Geometry: final body of the model. Coordinates: model frame, mm. Give positions to 0.01 mm unless a question says otherwise; leave off trailing zeros. Write each loop counter-clockwise with the first axis right and the second up, starting at its lowest first coordinate (ties: lowest second). Pieces come first, ordered by that corner, then holes.
Q1. Line query: line 1 (X direction, y = 0.15, z = -15); line 2 (X direction, y = -0.25, z = -17.25); line 3 (Z direction, x = 0.5, y = -0.05). Output: solid intervals per line, ascending.
Q2. Section C-C (y = -0.15). Return the cut outline in (x, z), plus the area to 3 significant figures.
Q3. Section A-A (x = 0). Return the cut outline in (y, z).
Q4. Section B-B (z = -17.5). Return the cut outline in (x, y), plus the area to 3 significant figures.
Q5. Mould query, pull axis Z, two halves, no side actions, for faces 1 (the cylindrical face through (0.16, -0.08, 7.5)), 2 (the flat face through (0, -1, -8)), 3 (the cylindrical face through (0.931, -0.083, 2.957)). Classes: +Z half, -Z half, draft (parallel to the pull), parting line (faces both ways), or undercut.
Q6. Section D-D (z = -2). Return the cut outline in (x, y).
from build123d import *

# Parameters (mm, degrees)
BOSS_EXTRUDE1_DEPTH      = 0.86
BOSS_EXTRUDE1_DEPTH_BACK = 1
SKETCH1_R                = 3.1


with BuildPart() as part:
    # Sketch1 → Boss-Extrude1 (new, two sides: drawn at the far end of the back side and taken through both)
    with BuildSketch(Plane(origin=(0, 0, 0), x_dir=(1, 0, 0), z_dir=(0, 1, 0)).offset(-BOSS_EXTRUDE1_DEPTH_BACK)):
        with BuildLine():
            Line((-7.5, 0), (-7.5, 15))
            ThreePointArc((-7.5, 15), (0, 22.5), (7.5, 15))
            Line((7.5, 15), (7.5, 0))
            ThreePointArc((7.5, 0), (0, -7.5), (-7.5, 0))
        make_face()
        with Locations(Location((0, 0, 0), (0, 0, 270))):
            Circle(SKETCH1_R, mode=Mode.SUBTRACT)
        with Locations(Location((0, 15, 0), (0, 0, 270))):
            Circle(SKETCH1_R, mode=Mode.SUBTRACT)
    extrude(amount=BOSS_EXTRUDE1_DEPTH + BOSS_EXTRUDE1_DEPTH_BACK)


solid = part.part
Computed:
1. line 1: x = -7.5 to -3.1, 3.1 to 7.5
1. line 2: x = -7.15 to -2.13, 2.13 to 7.15
1. line 3: z = -22.48 to -18.06, -11.94 to -3.06, 3.06 to 7.48
2. outline: (-7.5, -15) arc R7.5 ccw to (7.5, -15) - (7.5, 0) arc R7.5 ccw to (-7.5, 0) - close; hole circle Ø6.2 at (0, -15); hole circle Ø6.2 at (0, 0)
2. area: 341 mm2
3. outline: (-1, -22.5) - (0.86, -22.5) - (0.86, -18.1) - (-1, -18.1) - close; (-1, -11.9) - (0.86, -11.9) - (0.86, -3.1) - (-1, -3.1) - close; (-1, 3.1) - (0.86, 3.1) - (0.86, 7.5) - (-1, 7.5) - close
4. outline: (-7.07, -1) - (-1.83, -1) - (-1.83, 0.86) - (-7.07, 0.86) - close; (1.83, -1) - (7.07, -1) - (7.07, 0.86) - (1.83, 0.86) - close
4. area: 19.5 mm2
5. face 1: +Z half
5. face 2: draft
5. face 3: undercut
6. outline: (-7.5, -1) - (-2.37, -1) - (-2.37, 0.86) - (-7.5, 0.86) - close; (2.37, -1) - (7.5, -1) - (7.5, 0.86) - (2.37, 0.86) - close
